The listing builds one solid part. Answer for the finished solid, in the listing's coordinates (mm). Face numbers are marked on the shaded views. A direction names the side the tool comes from. Give positions to 0.01 mm unless a question says otherwise; leave off trailing zeros. Loops run counter-clockwise (first coordinate to the right, second up) from the corner with the lowest first, then second, coordinate; pieces in that order, holes last. Notation, with made-up numbers: M -38.75,82 L -5.75,82 A22 ccw -5.75,89 Z; hole C 1.25,78.5 d1. An arc over 180 degrees is marked long. Use one line per item in the form item = value. Start each with the question number.
1. For the marked faces 1, 2 and 3, determine the directions among +Z, -Z, +X, -X, +Y, -Y from which every point of the face is accessible in a straight line to the end or side of a thin tool.
2. The part is cut by section D-D (z = -17). Write down the section's boundary in (x, y), and give its area (3 significant figures).
3. The part is cut by section B-B (x = 14). Write down the section's boundary in (y, z), and give its area (3 significant figures).
4. The part is cut by section C-C (z = -1.5). Write down the section's boundary in (x, y).
5. Straight lines are drawn through the part: line 1 (Z direction, x = 21, y = -5); line 2 (X direction, y = -3.25, z = -14.5); line 3 (Z direction, x = 7, y = -7.5). For each, find the intervals that lie inside material, in ascending order. Write a range as from..to.
6. The part is cut by section A-A (y = -5). Write down the section's boundary in (x, z).
7. Each of these flat-tipped pins is pushed along its axis until it touches: pin 1 Ø1.5 at (x, y) = (-10.5, -4.5) entering from -Z; pin 2 Ø3 at (y, z) = (-3.5, -11) entering from -X. Where does it stop, or does it pass through?
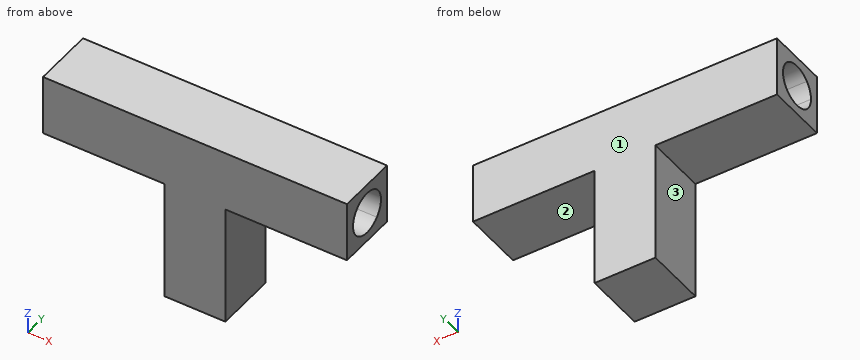
from build123d import *

# Parameters (mm, degrees)
F1_DEPTH = 10
F3_DEPTH = 50.001


with BuildPart() as f1:
    # F0 (on Front) → F1 (new body)
    with BuildSketch(Plane.XZ):
        Polygon((25, -5), (25, 5), (-25, 5), (-25, -5), (-5, -5), (-5, -25), (5, -25), (5, -5), align=None)
    extrude(amount=F1_DEPTH)

    # F2 (on face) → F3 (cut, through all)
    with BuildSketch(Plane(origin=(-25, 0, 0), x_dir=(0, -1, 0), z_dir=(-1, 0, 0))):
        with BuildLine():
            ThreePointArc((2.525126, -2.474874), (6.339392, -3.233578), (8.5, 0))
            ThreePointArc((8.5, 0), (8.233578, 1.339392), (7.474874, 2.474874))
            ThreePointArc((7.474874, 2.474874), (2.525126, 2.474874), (2.525126, -2.474874))
        make_face()
    extrude(amount=-F3_DEPTH, mode=Mode.SUBTRACT)


solid = f1.part
Derived:
q1.face_1 = +Z, -Z, +X, -X, +Y
q1.face_2 = -Z, +X, +Y, -Y
q1.face_3 = -Z, -X, +Y, -Y
q2.outline = M -5,-10 L 5,-10 L 5,0 L -5,0 Z
q2.area = 100 mm2
q3.outline = M -10,-5 L 0,-5 L 0,5 L -10,5 Z; hole M -8.5,0 A3.5 ccw long -7.47,2.47 A3.5 ccw Z
q3.area = 61.5 mm2
q4.outline = M -25,-10 L 25,-10 L 25,-8.16 L -25,-8.16 Z; M -25,-1.84 L 25,-1.84 L 25,0 L -25,0 Z
q5.line_1 = -5..-3.5, 3.5..5
q5.line_2 = -5..5
q5.line_3 = -5..-2.45, 2.45..5
q6.outline = M -25,-5 L -5,-5 L -5,-25 L 5,-25 L 5,-5 L 25,-5 L 25,-3.5 L -25,-3.5 Z; M -25,3.5 L 25,3.5 L 25,5 L -25,5 Z
q7.pin_1 = -5
q7.pin_2 = -5
